Design review of the part built by this model. Coordinates are the model's own, in mm. Face numbers are marked on the shaded views. A direction names the side the tool comes from. Coordinates: 2 decimals unless noted, no trailing zeros. Loops run counter-clockwise (first coordinate to the right, second up) from the corner with the lowest first, then second, coordinate; pieces in that order, holes last. Notation, with made-up numbers: M -40,20.25 L -34,20.25 A34 cw -34,54.25 Z; hole C 38,-3 d5. An arc over 180 degrees is marked long. Put each result on its own line as item: value. Start each with the question number.
(1) Clearance check with flat-ended pins moving along their axes: pin 1 (1.5 mm diameter, centred on y = 5, z = 8, fed in from -X); pin 2 (1 mm diameter, centred on x = 4.5, z = 8.5, fed in from -Y); pin 3 (6.5 mm diameter, centred on x = 0, y = 0, fed in from +Z); pin 4 (1 mm diameter, centred on x = -2, z = 4.5, fed in from -Y). State where each tip first meets the part, or that it passes through.
(2) Take a section at A-A, the plane y = 0. Give the boundary of the cut face in (x, z).
(3) Take a section at C-C, the plane z = 7.75. Give the boundary of the cut face in (x, y), then the cut area to 3 significant figures.
(4) Take a section at D-D, the plane z = 3.5. Give the boundary of the cut face in (x, y).
(5) For the marked faces 1 and 2, list the 3-axis set-ups (+Z, -Z, +X, -X, +Y, -Y) from which the entire face can be reached by the end or side of a thin tool; tool diameter is ignored.
(6) For probe 1 along Z at (x, y) = (0, -6.4); probe 2 along Y at (x, z) = (-2.25, 5.75); probe 3 along X at (y, z) = (-3.25, 6.5), list the stretches that pass through material, from the lowest coordinate up. Write a range as [from, to].
(7) Take a section at B-B, the plane x = 0. Give the boundary of the cut face in (y, z).
(8) The part is to be moulded in two halves that separate along X. For the marked faces 3, 4 and 5, say which applies: +X half, -X half, draft (parallel to the pull), parting line (faces both ways), or undercut.
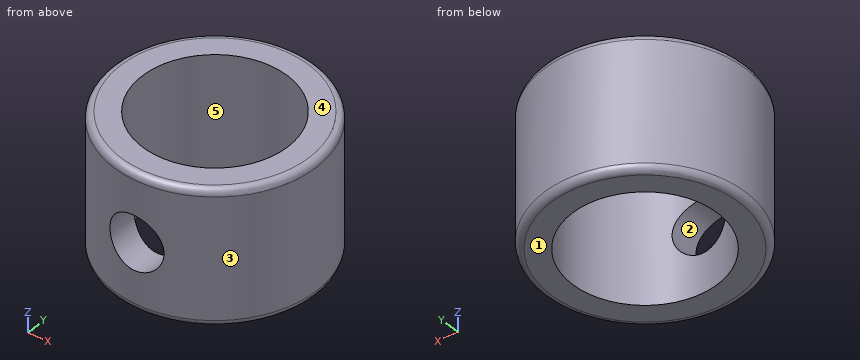
Autodesk Inventor part; units mm, degrees
ref_plane "YZ Plane" through (0, 0, 0) normal (1, 0, 0) x (0, 1, 0)
ref_plane "XZ Plane" through (0, 0, 0) normal (0, 1, 0) x (-1, 0, 0)
ref_plane "XY Plane" through (0, 0, 0) normal (0, 0, 1) x (1, 0, 0)
sketch "Sketch1" plane through (0, 0, 0) normal (0, 0, 1) x (1, 0, 0)
  circle A0 centre (0, 0) radius 5.4
  circle A1 centre (0, 0) radius 7.5
  dimension "d0" = 10.8
  dimension "d1" = 15
extrude "Extrusion1" add sketch "Sketch1" along normal blind 10
fillet "Fillet1" radius 0.5 2 edges at (-7.5, 0, 10) (-7.5, 0, 0)
sketch "Sketch4" plane through (0, 0, 0) normal (0, 1, 0) x (-1, 0, 0)
  circle A0 centre (0, 4.9172) radius 2
  point P0 (0, 0)
  dimension "d5" = 4
extrude "Extrusion2" cut sketch "Sketch4" against normal blind 10
equation "\"BendRadius\" = Thickness"
equation "\"BendReliefWidth\" = Thickness"
equation "\"BendReliefDepth\" = 0.5 * Thickness"
equation "\"CornerReliefSize\" = 4 * Thickness"
equation "\"MinimumRemnant\" = 2 * Thickness"
equation "\"TransitionRadius\" = BendRadius"
equation "\"JacobiRadiusSize\" = BendRadius"
equation "\"GapSize\" = Thickness"
properties part number "khóa trục"
Computed values:
1. pin 1: stops at x = -6.18
1. pin 2: stops at y = -6.34
1. pin 3: passes through
1. pin 4: stops at y = -7.28
2. outline: M -7.5,0.5 A0.5 ccw -7,0 L -5.4,0 L -5.4,10 L -7,10 A0.5 ccw -7.5,9.5 Z; M 5.4,0 L 7,0 A0.5 ccw 7.5,0.5 L 7.5,9.5 A0.5 ccw 7,10 L 5.4,10 Z
3. outline: C 0,0 d15; hole C 0,0 d10.8
3. area: 85.1 mm^2
4. outline: M -1.41,-7.37 L -1.41,-5.21 A5.4 cw long 1.41,-5.21 L 1.41,-7.37 A7.5 ccw long Z
5. face 1: -Z, +X, -X, +Y, -Y
5. face 2: -Y
6. probe 1: z = [0, 2.92], [6.92, 10]
6. probe 2: y = [-7.15, -4.91], [4.91, 7.15]
6. probe 3: x = [-6.76, -4.31], [4.31, 6.76]
7. outline: M -7.5,0.5 A0.5 ccw -7,0 L -5.4,0 L -5.4,2.92 L -7.5,2.92 Z; M -7.5,6.92 L -5.4,6.92 L -5.4,10 L -7,10 A0.5 ccw -7.5,9.5 Z; M 5.4,0 L 7,0 A0.5 ccw 7.5,0.5 L 7.5,9.5 A0.5 ccw 7,10 L 5.4,10 Z
8. face 3: parting line
8. face 4: draft
8. face 5: undercut
